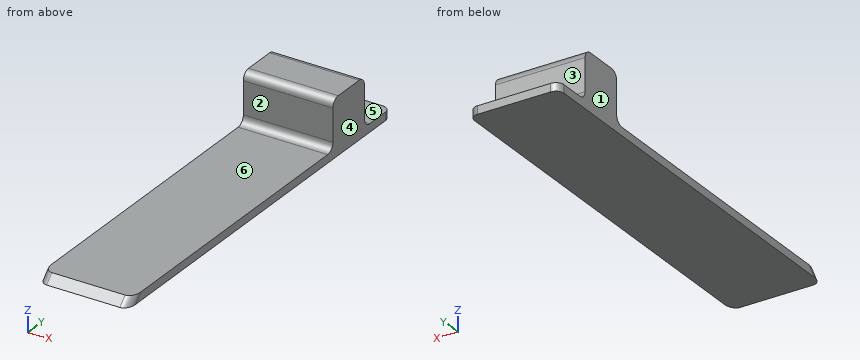
```python
from build123d import *

# Parameters (mm, degrees)
SZKIC1_W                    = 11
SZKIC1_H                    = 50
DODANIE_WYCI_GNI_CIE1_DEPTH = 1
SFAZOWANIE1_SIZE            = 1
SZKIC2_W                    = 11
SZKIC2_H                    = 6
DODANIE_WYCI_GNI_CIE2_DEPTH = 6
ZAOKR_GLENIE1_R             = 1


with BuildPart() as part:
    # Szkic1 → Dodanie-wyciągnięcie1 (new body)
    with BuildSketch(Plane.XY):
        Rectangle(SZKIC1_W, SZKIC1_H)
    extrude(amount=DODANIE_WYCI_GNI_CIE1_DEPTH)

    # Sfazowanie1
    sfazowanie1_edges = [part.edges().sort_by_distance(p)[0] for p in [
        (0, -25, 1),
    ]]
    chamfer(sfazowanie1_edges, length=SFAZOWANIE1_SIZE - 0.0001)  # a hair under: the kernel refuses the full size

    # Szkic2 → Dodanie-wyciągnięcie2 (add)
    with BuildSketch(Plane.XY.offset(1)):
        with Locations((0, 17)):
            Rectangle(SZKIC2_W, SZKIC2_H)
    extrude(amount=DODANIE_WYCI_GNI_CIE2_DEPTH)

    # Zaokrąglenie1
    zaokr_glenie1_edges = [part.edges().sort_by_distance(p)[0] for p in [
        (5.5, -24.50005, 0.50005),
        (-5.5, -24.50005, 0.50005),
        (0, 14, 1),
        (0, 20, 1),
        (0, 14, 7),
        (0, 20, 7),
        (-5.5, 25, 0.5),
        (5.5, 25, 0.5),
    ]]
    fillet(zaokr_glenie1_edges, radius=ZAOKR_GLENIE1_R)


solid = part.part
```
Geometry: final body of the model. Coordinates: model frame, mm. Face numbers are marked on the shaded views. A direction names the side the tool comes from. Coordinates: 2 decimals unless noted, no trailing zeros. Order: outer loops, then holes, each group sorted by start corner. A loop starts at its lowest first (then second) coordinate and runs counter-clockwise, first axis right, second up. Notation, with made-up numbers: (-11.75, 66) -> (39.25, 66) arc R18 ccw to (39.25, 74) -> close; hole circle Ø3 at (87, 42). An arc over 180 degrees is marked (long way). Write item = value, one per line.
(1) Cut plane C-C on y = -15. Return loops of the section in (x, z), plus the area to 3 significant figures.
Solved:
outline = (-5.5, 0) -> (5.5, 0) -> (5.5, 1) -> (-5.5, 1) -> close
area = 11.0 mm²
(2) Access query for the marked faces 4, 5 and 6. Directions: +Z, -Z, +X, -X, +Y, -Y. A direction counts if a zero-diameter tool reaches every point of the face in a straight line with its end or side. Return the directions, or none.
Solved:
face_4 = +Z, -Z, +X, +Y, -Y
face_5 = +Z, +X, -X, +Y
face_6 = +Z, +X, -X, -Y
(3) Pull-direction query (Y, two-part tool) for the marked faces 1, 2 and 3; classes: pulls with the +Y half, pulls with the -Y half, needs draft (parallel to the pull), parting line crosses it, or undercut.
Solved:
face_1 = needs draft
face_2 = pulls with the -Y half
face_3 = pulls with the +Y half
(4) Line query: line 1 (Z direction, x = 4.75, y = -21); line 2 (Y direction, x = -3.25, z = 6); line 3 (Y direction, x = 1, z = 0.5). Output: solid intervals per line, ascending.
Solved:
line_1 = 0 to 1
line_2 = 14 to 20
line_3 = -24.5 to 25
(5) Cut plane B-B on z = 4.5. Return loops of the section in (x, y).
Solved:
outline = (-5.5, 14) -> (5.5, 14) -> (5.5, 20) -> (-5.5, 20) -> close
(6) Pin query (flat end, axial travel): pin 1 Ø1.5 at (x, y) = (0, 1) entering from +Z; pin 2 Ø4 at (y, z) = (-6, 3.5) entering from -X; pin 3 Ø2 at (x, z) = (-1, 3.5) entering from -Y; pin 4 Ø2 at (x, z) = (-4, 4.5) entering from +Y. Return the tip coordinate at first contact, or that it passes through.
Solved:
pin_1 = 1
pin_2 = through
pin_3 = 14
pin_4 = 20
